Geometry: final body of the model. Coordinates: model frame, mm. Face numbers are marked on the shaded views. Give positions to 0.01 mm unless a question says otherwise; leave off trailing zeros. Loops run counter-clockwise (first coordinate to the right, second up) from the corner with the lowest first, then second, coordinate; pieces in that order, holes last.
from build123d import *

# Parameters (mm, degrees)
RESSALTO_EXTRUS_O1_DEPTH      = 5
RESSALTO_EXTRUS_O1_DEPTH_BACK = 5
CORTE_EXTRUS_O1_DEPTH         = 5
CORTE_EXTRUS_O1_DEPTH_BACK    = 5
ESBO_O1_R                     = 4
ESBO_O1_R_2                   = 2.5


with BuildPart() as part:
    # Esbo_o2 → Ressalto-extrus_o1 (new, two sides: drawn at the far end of the back side and taken through both)
    with BuildSketch(Plane(origin=(0, 0, 0), x_dir=(1, 0, 0), z_dir=(0, 1, 0)).offset(-RESSALTO_EXTRUS_O1_DEPTH_BACK)):
        with BuildLine():
            Line((16, 10), (-16, 10))
            ThreePointArc((-16, 10), (-26, 0), (-16, -10))
            Line((-16, -10), (16, -10))
            ThreePointArc((16, -10), (26, 0), (16, 10))
        make_face()
    extrude(amount=RESSALTO_EXTRUS_O1_DEPTH + RESSALTO_EXTRUS_O1_DEPTH_BACK)

    # Esbo_o1 → Corte-extrus_o1 (cut, two sides: drawn at the far end of the back side and taken through both)
    with BuildSketch(Plane(origin=(0, 0, 0), x_dir=(1, 0, 0), z_dir=(0, 1, 0)).offset(-CORTE_EXTRUS_O1_DEPTH_BACK)):
        with Locations(Location((0, 0, 0), (0, 0, 270))):
            Circle(ESBO_O1_R)
        with Locations(Location((16, 0, 0), (0, 0, 270))):
            Circle(ESBO_O1_R_2)
        with Locations(Location((-16, 0, 0), (0, 0, 270))):
            Circle(ESBO_O1_R_2)
    extrude(amount=CORTE_EXTRUS_O1_DEPTH + CORTE_EXTRUS_O1_DEPTH_BACK, mode=Mode.SUBTRACT)


solid = part.part
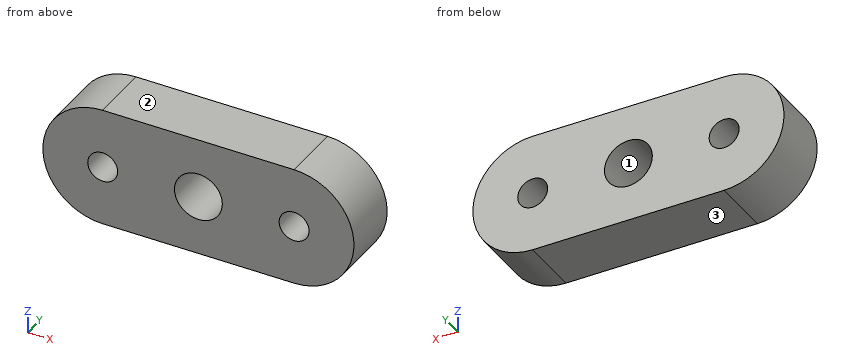
Item 1: Section query C-C on z = 0.5. Return loops of the section in (x, y).
Values follow:
outline: (-25.99, -5) - (-18.45, -5) - (-18.45, 5) - (-25.99, 5) - close; (-13.55, -5) - (-3.97, -5) - (-3.97, 5) - (-13.55, 5) - close; (3.97, -5) - (13.55, -5) - (13.55, 5) - (3.97, 5) - close; (18.45, -5) - (25.99, -5) - (25.99, 5) - (18.45, 5) - close
Item 2: Section query B-B on z = 3.5. Return loops of the section in (x, y), plus the area to 3 significant figures.
Values follow:
outline: (-25.37, -5) - (-1.94, -5) - (-1.94, 5) - (-25.37, 5) - close; (1.94, -5) - (25.37, -5) - (25.37, 5) - (1.94, 5) - close
area: 469 mm2
Item 3: Draft query along Z for the marked faces 1, 2 and 3. Return one class per face: +Z half, -Z half, draft (parallel to the pull), parting line (faces both ways), or undercut.
Values follow:
face 1: undercut
face 2: +Z half
face 3: -Z half
Item 4: Pin query (flat end, axial travel): pin 1 (6 mm diameter, centred on y = 3.5, z = -4, fed in from +X); pin 2 (5 mm diameter, centred on y = -3, z = -5, fed in from +X); pin 3 (2 mm diameter, centred on y = 1, z = -7, fed in from +X). Return the tip coordinate at first contact, or that it passes through.
Values follow:
pin 1: stops at x = 25.95
pin 2: stops at x = 25.68
pin 3: stops at x = 24
Item 5: Section query D-D on x = -18. Return loops of the section in (y, z).
Values follow:
outline: (-5, -9.8) - (5, -9.8) - (5, -1.5) - (-5, -1.5) - close; (-5, 1.5) - (5, 1.5) - (5, 9.8) - (-5, 9.8) - close
Item 6: Ray query, probe 1 along X at (y, z) = (0.75, 0); probe 2 along X at (y, z) = (0.5, 1.75); probe 3 along Z at (x, y) = (-17, -3.25). Return the intervals inside material, ascending.
Values follow:
probe 1: x = -26 to -18.5, -13.5 to -4, 4 to 13.5, 18.5 to 26
probe 2: x = -25.85 to -17.79, -14.21 to -3.6, 3.6 to 14.21, 17.79 to 25.85
probe 3: z = -9.95 to -2.29, 2.29 to 9.95
Item 7: Section query A-A on y = -3. Return loops of the section in (x, z).
Values follow:
outline: (-16, -10) - (16, -10) arc R10 ccw to (16, 10) - (-16, 10) arc R10 ccw to start; hole circle Ø5 at (-16, 0); hole circle Ø8 at (0, 0); hole circle Ø5 at (16, 0)
